from build123d import *

# Parameters (mm, degrees)
BOSS_EXTRUDE1_DEPTH = 3.175


with BuildPart() as part:
    # Sketch1 → Boss-Extrude1 (new body)
    with BuildSketch(Plane(origin=(0, 0, 0), x_dir=(1, 0, 0), z_dir=(0, 1, 0))):
        Polygon((-39.972456053, 57.15), (173.151878886, 57.15), (133.179422833, 0), (0, 0), align=None)
        Polygon((-18.245720617, 42.70524807), (-14.606223674, 37.50173368), (-17.207980869, 35.681985209), (-20.847477812, 40.885499598), align=None, mode=Mode.SUBTRACT)
        Polygon((-10.966726732, 32.29821929), (-13.568483927, 30.478470819), (-9.928986984, 25.274956429), (-7.327229789, 27.0947049), align=None, mode=Mode.SUBTRACT)
        Polygon((-0.048235904, 16.687676121), (-2.649993099, 14.867927649), (-6.289490041, 20.071442039), (-3.687732847, 21.89119051), align=None, mode=Mode.SUBTRACT)
        Polygon((3.591261039, 11.484161731), (0.989503844, 9.66441326), (4.629000786, 4.46089887), (7.230757981, 6.280647341), align=None, mode=Mode.SUBTRACT)
        Polygon((155.064640392, 47.908762459), (157.666397587, 46.089013988), (161.30589453, 51.292528378), (158.704137335, 53.112276849), align=None, mode=Mode.SUBTRACT)
        Polygon((125.948664851, 6.280647341), (129.588161794, 11.484161731), (132.189918989, 9.66441326), (128.550422046, 4.46089887), align=None, mode=Mode.SUBTRACT)
        Polygon((139.468912874, 20.071442039), (135.829415932, 14.867927649), (133.227658737, 16.687676121), (136.867155679, 21.89119051), align=None, mode=Mode.SUBTRACT)
        Polygon((140.506652622, 27.0947049), (144.146149564, 32.29821929), (146.747906759, 30.478470819), (143.108409817, 25.274956429), align=None, mode=Mode.SUBTRACT)
        Polygon((-25.524714502, 53.112276849), (-21.88521756, 47.908762459), (-24.486974754, 46.089013988), (-28.126471697, 51.292528378), align=None, mode=Mode.SUBTRACT)
        Polygon((147.785646507, 37.50173368), (150.387403702, 35.681985209), (154.026900645, 40.885499598), (151.42514345, 42.70524807), align=None, mode=Mode.SUBTRACT)
    extrude(amount=BOSS_EXTRUDE1_DEPTH)


solid = part.part
Check sheet for the modelled part. Datum: model origin and axes. Units: mm. A direction names the side the tool comes from. Give positions to 0.01 mm unless a question says otherwise; leave off trailing zeros. Use a Markdown table: item, result. Add a question column.
Q1. Mould release check, pull along Z, two halves, no side actions. Record for faces 3 (the flat face through (68, 3.175, -29)), 4 (the flat face through (-16.45, 1.57, -40.14)), 5 (the flat face through (-1.893, 1.565, -19.326)), 6 (the flat face through (153.45, 1.57, -28.98)): pulls with the +Z half, pulls with the -Z half, needs draft (parallel to the pull), parting line crosses it, or undercut.
Q2. Sectioned sample at A-A, the plane y = 0.5. Give the number of separate pieces and of enclosed holes in the cut face, then the cut area to 3 significant figures.
Q3. Go/stop test with flat-tipped pins: pin 1 (1 mm diameter, centred on y = 1, z = -20, fed in from -X); pin 2 (1 mm diameter, centred on y = 1, z = -18.5, fed in from +X). Record where each tip stops, or that it passes through.
Q4. Tool access check on faces 1 (the flat face through (2.784, 1.565, -7.099)), 2 (the flat face through (68, 0, -29)). Record the directions out of +Z, -Z, +X, -X, +Y, -Y that give a thin tool (end or side, any length) a straight path to the whole face; none if there is none.
Q5. Scan lines: line 1 along X through (y, z) = (1.25, -19); line 2 along X through (y, z) = (0.45, -37); line 3 along Z through (x, y) = (-22, 0.45). Record each from-to range of solid material in increasing order. Write a range as [from, to].
Verdict:
| question | item | result |
|---|---|---|
| 1 | face 3 | needs draft |
| 1 | face 4 | undercut |
| 1 | face 5 | undercut |
| 1 | face 6 | pulls with the +Z half |
| 2 | separate pieces | 1 |
| 2 | enclosed holes | 10 |
| 2 | area | 9,690 mm^2 |
| 3 | pin 1 | x = -14.34 |
| 3 | pin 2 | x = 146.47 |
| 4 | face 1 | +Y, -Y |
| 4 | face 2 | +Z, -Z, +X, -X, -Y |
| 5 | line 1 | [-13.29, -5.54], [-1.67, 134.84], [138.72, 146.47] |
| 5 | line 2 | [-25.88, -18.13], [-15.32, 148.5], [151.31, 159.06] |
| 5 | line 3 | [-57.15, -48.07], [-47.83, -31.45] |
